Verification items for the finished model (mm, model axes). A direction names the side the tool comes from. Coordinates: 2 decimals unless noted, no trailing zeros. Order: outer loops, then holes, each group sorted by start corner. A loop starts at its lowest first (then second) coordinate and runs counter-clockwise, first axis right, second up.
Q1. Set-up check for faces 1 (the cylindrical face through (12.417, 55.918, -61.971)), 2 (the cylindrical face through (62.44, -2.75, -60.29)), 3 (the cylindrical face through (19.238, -146.522, 113.029)): record each of +Z, -Z, +X, -X, +Y, -Y from which the full face is reachable in a straight line by a thin tool's end or side.
Q2. Cross-section at A-A, the plane x = 0. Record the boundary of the cut face in (y, z).
Q3. Cross-section at D-D, the plane z = 25. Record the boundary of the cut face in (x, y).
Q4. Cross-section at C-C, the plane z = 110. Record the boundary of the cut face in (x, y), and give its area (3 significant figures).
Q5. Depth check by flat-ended pin: P1, Ø8, axis at x = 75.5, y = 99, coming from the -Z side; P2, Ø10, axis at x = 104.5, y = 12.5, coming from the +Z side; P3, Ø4, axis at y = -106.5, z = 54.5, coming from the -X side. Enter the tip coordinate at first touch or a pass-through.
Q6. Draft check along Y on faces 4 (the flat face through (-39, 43, -74.646)), 5 (the conical face through (-39.699, -62.266, -9.681)), 6 (the conical face through (46.58, 35.71, -74.45)). Enter one of: pulls with the +Y half, pulls with the -Y half, needs draft (parallel to the pull), parting line crosses it, or undercut.
Q7. Thickness scan on line 1 (Y direction, x = 0, z = 118); line 2 (X direction, y = 0, z = -60.5). Record the ranges inside material, lowest first.
from build123d import *

# Parameters (mm, degrees)
F2_SIZE = 4


with BuildPart() as f1:
    # F0 (on Front) → F1 (revolve)
    with BuildSketch(Plane.XZ):
        with BuildLine():
            Line((-147.78, 125.353982), (-153, 125.353982))
            Line((-153, 125.353982), (-153, 100.353982))
            ThreePointArc((-153, 100.353982), (-149.515286, 80.203983), (-139.465919, 62.394551))
            Line((-139.465919, 62.394551), (-73.778401, -18.01316))
            ThreePointArc((-73.778401, -18.01316), (-65.403928, -32.854353), (-62.5, -49.646018))
            Line((-62.5, -49.646018), (-62.5, -74.646018))
            Line((-62.5, -74.646018), (-57.28, -74.646018))
            Line((-57.28, -74.646018), (-57.28, -49.646018))
            ThreePointArc((-57.28, -49.646018), (-60.487098, -31.101303), (-69.735866, -14.710689))
            Line((-69.735866, -14.710689), (-135.423384, 65.697021))
            ThreePointArc((-135.423384, 65.697021), (-144.598456, 81.957033), (-147.78, 100.353982))
            Line((-147.78, 100.353982), (-147.78, 125.353982))
        make_face()
    revolve(axis=Axis((0, 0, 32.767496), (0, 0, 1)))

    # F2
    f2_edges = [f1.edges().sort_by_distance(p)[0] for p in [
        (153, 0, 125.353982),
        (62.5, 0, -74.646018),
    ]]
    chamfer(f2_edges, length=F2_SIZE)


solid = f1.part
Check values:
1. face 1: +Z, -Z
1. face 2: -Z
1. face 3: +Z
2. outline: (-153, 100.35) arc R60 ccw to (-139.47, 62.39) - (-73.78, -18.01) arc R50 cw to (-62.5, -49.65) - (-62.5, -70.65) - (-58.5, -74.65) - (-57.28, -74.65) - (-57.28, -49.65) arc R55.22 ccw to (-69.74, -14.71) - (-135.42, 65.7) arc R54.78 cw to (-147.78, 100.35) - (-147.78, 125.35) - (-149, 125.35) - (-153, 121.35) - close; (57.28, -74.65) - (58.5, -74.65) - (62.5, -70.65) - (62.5, -49.65) arc R50 cw to (73.78, -18.01) - (139.47, 62.39) arc R60 ccw to (153, 100.35) - (153, 121.35) - (149, 125.35) - (147.78, 125.35) - (147.78, 100.35) arc R54.78 cw to (135.42, 65.7) - (69.74, -14.71) arc R55.22 ccw to (57.28, -49.65) - close
3. outline: circle Ø217.83 at (0, 0); hole circle Ø204.35 at (0, 0)
4. outline: circle Ø306 at (0, 0); hole circle Ø295.56 at (0, 0)
4. area: 4,930 mm2
5. P1: stops at z = 39.18
5. P2: stops at z = 34.88
5. P3: stops at x = -83.42
6. face 4: needs draft
6. face 5: undercut
6. face 6: parting line crosses it
7. line 1: y = -153 to -147.78, 147.78 to 153
7. line 2: x = -62.5 to -57.28, 57.28 to 62.5
